Design review of the part built by this model. Coordinates are the model's own, in mm. Round coordinates to 2 decimals unless told otherwise and drop trailing zeros. Loops run counter-clockwise (first coordinate to the right, second up) from the corner with the lowest first, then second, coordinate; pieces in that order, holes last. Notation, with made-up numbers: (-34.75, -15.75) - (-12.75, -15.75) arc R10 cw to (-12.75, -1.75) - close; hole circle Ø2 at (21.5, 32). An arc over 180 degrees is marked (long way). Return JSON: item names as keys, results as strings. Group by question number.
Autodesk Inventor part; units mm, degrees
ref_plane "YZ Plane" through (0, 0, 0) normal (1, 0, 0) x (0, 1, 0)
ref_plane "XZ Plane" through (0, 0, 0) normal (0, 1, 0) x (-1, 0, 0)
ref_plane "XY Plane" through (0, 0, 0) normal (0, 0, 1) x (1, 0, 0)
sketch "Эскиз1" plane through (0, 0, 0) normal (0, 0, 1) x (1, 0, 0)
  line L0 (-20, -22.5) -> (-20, -19.5)
  line L1 (-20, -19.5) -> (-30, -19.5)
  line L2 (-30, -19.5) -> (-30, -22.5)
  line L3 (0, -19.5) -> (-5, -19.5)
  line L4 (-5, -19.5) -> (-5, -22.5)
  line L5 (20, -22.5) -> (20, -19.5)
  line L6 (20, -19.5) -> (30, -19.5)
  line L7 (30, -19.5) -> (30, -22.5)
  line L8 (0, -19.5) -> (5, -19.5)
  line L9 (5, -19.5) -> (5, -22.5)
  line L10 (-53, 22.5) -> (-30, 22.5)
  line L11 (-20, 22.5) -> (-20, 19.5)
  line L12 (-20, 19.5) -> (-30, 19.5)
  line L13 (-30, 19.5) -> (-30, 22.5)
  line L14 (-20, 22.5) -> (-5, 22.5)
  line L15 (0, 19.5) -> (-5, 19.5)
  line L16 (-5, 19.5) -> (-5, 22.5)
  line L17 (-5, 22.5) -> (-20, 22.5)
  line L18 (-30, 22.5) -> (-53, 22.5)
  line L19 (53, 22.5) -> (30, 22.5)
  line L20 (20, 22.5) -> (20, 19.5)
  line L21 (20, 19.5) -> (30, 19.5)
  line L22 (30, 19.5) -> (30, 22.5)
  line L23 (20, 22.5) -> (5, 22.5)
  line L24 (0, 19.5) -> (5, 19.5)
  line L25 (5, 19.5) -> (5, 22.5)
  line L26 (5, 22.5) -> (20, 22.5)
  line L27 (30, 22.5) -> (53, 22.5)
  line L28 (-20, -32.5) -> (-20, -29.5)
  line L29 (-20, -29.5) -> (-30, -29.5)
  line L30 (-30, -29.5) -> (-30, -32.5)
  line L31 (5, -32.5) -> (5, -29.5)
  line L32 (5, -29.5) -> (-5, -29.5)
  line L33 (-5, -29.5) -> (-5, -32.5)
  line L34 (30, -32.5) -> (30, -29.5)
  line L35 (30, -29.5) -> (20, -29.5)
  line L36 (20, -29.5) -> (20, -32.5)
  line L37 (-30, -22.5) -> (-20, -22.5)
  line L38 (-5, -22.5) -> (5, -22.5)
  line L39 (20, -22.5) -> (30, -22.5)
  line L40 (-30, -32.5) -> (-53, -32.5)
  line L41 (-5, -32.5) -> (-20, -32.5)
  line L42 (53, -32.5) -> (30, -32.5)
  line L43 (20, -32.5) -> (5, -32.5)
  line L44 (-53, 2.5) -> (-50, 2.5)
  line L45 (-50, 2.5) -> (-50, -12.5)
  line L46 (-50, -12.5) -> (-53, -12.5)
  line L47 (53, 2.5) -> (50, 2.5)
  line L48 (50, 2.5) -> (50, -12.5)
  line L49 (50, -12.5) -> (53, -12.5)
  line L50 (-53, 22.5) -> (-53, 2.5)
  line L51 (-53, -12.5) -> (-53, -32.5)
  line L52 (53, -32.5) -> (53, -12.5)
  line L53 (53, 2.5) -> (53, 22.5)
  circle A0 centre (0, 0) radius 3
  dimension "d15" = 6
extrude "Выдавливание1" add sketch "Эскиз1" along normal blind 3
properties part number "Стенка t2"
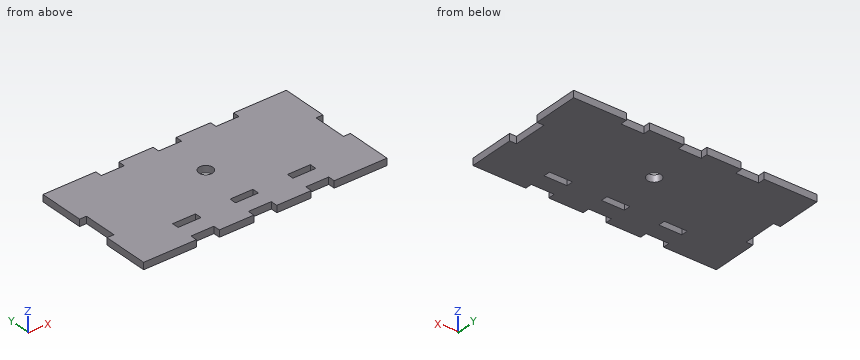
Q1. For line 1 (Y direction, x = 0, z = 1.7); line 2 (Y direction, x = 1, z = 2.4); line 3 (X direction, y = -10.5, z = 0.7), list the stretches that pass through material, from the lowest coordinate up.
Q2. Add section A-A, the plane x = 0. State the section outline as (y, z) points, plus the area to 3 significant figures.
Q3. Add section C-C, the plane z = 1.3. Give the number of separate pieces and of enclosed holes in the cut face, plus the area to 3 significant figures.
Q4. Insertion check: pin 1 Ø1.5 at (y, z) = (-4, 1.5) entering from +X; pin 2 Ø1.5 at (x, z) = (-0.5, 2) entering from -Y; pin 3 Ø1.5 at (x, z) = (27.5, 1) entering from +Y. Each pin has a flat end and moves straight along its axis. Give the tip position at first contact, or say it passes through.
Q5. Add section B-B, the plane y = 0. State the section outline as (x, z) points, plus the area to 3 significant figures.
Evaluation:
{
 "1": {"line 1": "-29.5 to -22.5, -19.5 to -3, 3 to 19.5", "line 2": "-29.5 to -22.5, -19.5 to -2.83, 2.83 to 19.5", "line 3": "-50 to 50"},
 "2": {"outline": "(-29.5, 0) - (-22.5, 0) - (-22.5, 3) - (-29.5, 3) - close; (-19.5, 0) - (-3, 0) - (-3, 3) - (-19.5, 3) - close; (3, 0) - (19.5, 0) - (19.5, 3) - (3, 3) - close", "area": "120 mm²"},
 "3": {"separate pieces": "1", "enclosed holes": "4", "area": "5,440 mm²"},
 "4": {"pin 1": "x = 50", "pin 2": "y = -29.5", "pin 3": "y = 19.5"},
 "5": {"outline": "(-50, 0) - (-3, 0) - (-3, 3) - (-50, 3) - close; (3, 0) - (50, 0) - (50, 3) - (3, 3) - close", "area": "282 mm²"}
}
